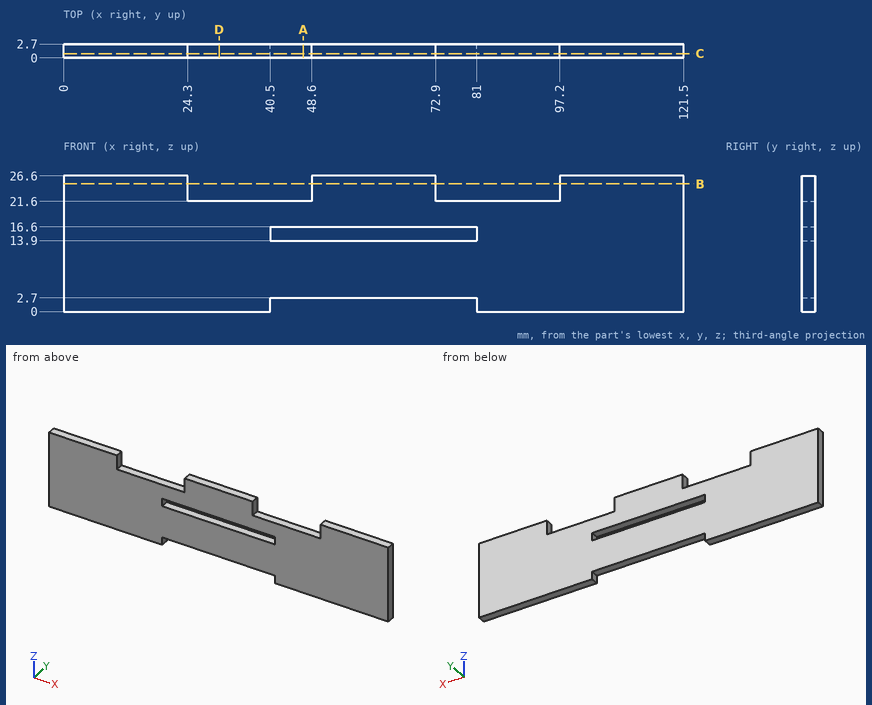
Answer from the drawing. Dimensions are ordinates in mm from the lowest x, y and z of the part. Coordinates: 2 decimals unless noted, no trailing zeros. Order: outer loops, then holes, each group sorted by start corner. A loop starts at its lowest first (then second) coordinate and runs counter-clockwise, first axis right, second up. Notation, with made-up numbers: (2.25, 62.5) - (40.25, 62.5) arc R35 ccw to (40.25, 97.5) - close; hole circle Ø7 at (29.25, -23.75). An arc over 180 degrees is marked (long way). Use one line per item in the form item = value.
(1) Section D-D, the plane x = 30.5 is taken. Give the vertices of the cut face in (y, z).
Computed values:
outline = (0, 0) - (2.7, 0) - (2.7, 21.6) - (0, 21.6) - close
(2) Given pin 1 Ø1.4 at (y, z) = (2, 23.5) entering from -X; pin 2 Ø0.8 at (x, y) = (33, 1.5) entering from +Z, each flat-ended and moving along its own axis, determine where each tip first touches the part or whether it passes through.
Computed values:
pin_1 = 0
pin_2 = 21.6
(3) Section A-A, the plane x = 47 is taken. Give the vertices of the cut face in (y, z), then the cut area to 3 significant figures.
Computed values:
outline = (0, 2.7) - (2.7, 2.7) - (2.7, 13.9) - (0, 13.9) - close; (0, 16.6) - (2.7, 16.6) - (2.7, 21.6) - (0, 21.6) - close
area = 43.7 mm²
(4) Section C-C, the plane y = 0.8 is taken. Give the vertices of the cut face in (x, z), then the cut area to 3 significant figures.
Computed values:
outline = (0, 0) - (40.5, 0) - (40.5, 2.7) - (81, 2.7) - (81, 0) - (121.5, 0) - (121.5, 26.6) - (97.2, 26.6) - (97.2, 21.6) - (72.9, 21.6) - (72.9, 26.6) - (48.6, 26.6) - (48.6, 21.6) - (24.3, 21.6) - (24.3, 26.6) - (0, 26.6) - close; hole (40.5, 13.9) - (81, 13.9) - (81, 16.6) - (40.5, 16.6) - close
area = 2,770 mm²
(5) Straight lines are drawn through the part: L1, parallel to Z at x = 72, y = 1.85; L2, parallel to X at y = 1.25, z = 23.5; L3, parallel to Z at x = 78, y = 1.15. For each, find the intervals that lie inside material, in ascending order.
Computed values:
L1 = 2.7 to 13.9, 16.6 to 26.6
L2 = 0 to 24.3, 48.6 to 72.9, 97.2 to 121.5
L3 = 2.7 to 13.9, 16.6 to 21.6
(6) Section B-B, the plane z = 25 is taken. Give the vertices of the cut face in (x, y), then the cut area to 3 significant figures.
Computed values:
outline = (0, 0) - (24.3, 0) - (24.3, 2.7) - (0, 2.7) - close; (48.6, 0) - (72.9, 0) - (72.9, 2.7) - (48.6, 2.7) - close; (97.2, 0) - (121.5, 0) - (121.5, 2.7) - (97.2, 2.7) - close
area = 197 mm²
